Input: dimensioned drawing with shaded views. Units: mm. Origin: part minimum x, y, z. Coordinates: 2 decimals unless noted, no trailing zeros. Loops run counter-clockwise (first coordinate to the right, second up) from the corner with the lowest first, then second, coordinate; pieces in that order, holes last.
Item 1: Pull-direction query (X, two-part tool) for the marked faces 1, 2 and 3; classes: +X half, -X half, draft (parallel to the pull), parting line (faces both ways), or undercut.
Item 2: Line query: probe 1 along Y at (x, z) = (127.5, 7.25); probe 2 along Y at (x, z) = (75, 15.5); probe 3 along X at (y, z) = (50, 4). Output: solid intervals per line, ascending.
Item 3: Section query D-D, the plane y = 47.5. Return the cut outline in (x, z), then the cut area to 3 significant figures.
Item 4: Section query B-B, the plane y = 20. Return the cut outline in (x, z).
Item 5: Section query C-C, the plane z = 11.25. Return the cut outline in (x, y), then the cut area to 3 significant figures.
Item 6: Section query A-A, the plane x = 75. Return the cut outline in (y, z), then the cut area to 3 significant figures.
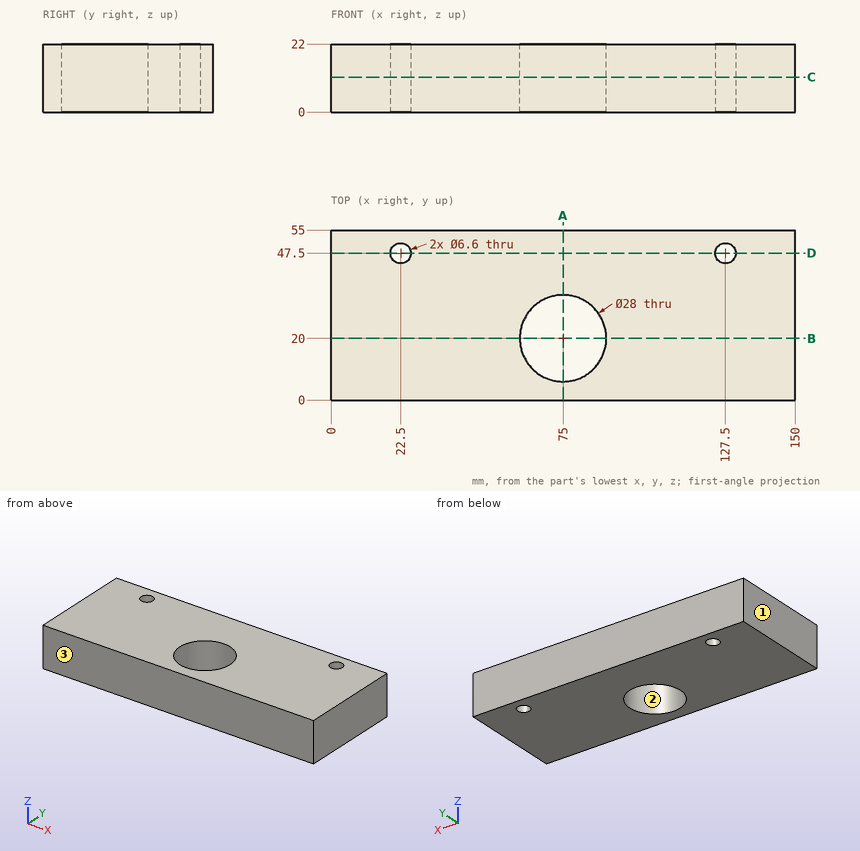
Verdict:
1. face 1: -X half
1. face 2: undercut
1. face 3: draft
2. probe 1: y = 0 to 44.2, 50.8 to 55
2. probe 2: y = 0 to 6, 34 to 55
2. probe 3: x = 0 to 20.35, 24.65 to 125.35, 129.65 to 150
3. outline: (0, 0) - (19.2, 0) - (19.2, 22) - (0, 22) - close; (25.8, 0) - (124.2, 0) - (124.2, 22) - (25.8, 22) - close; (130.8, 0) - (150, 0) - (150, 22) - (130.8, 22) - close
3. area: 3,010 mm2
4. outline: (0, 0) - (61, 0) - (61, 22) - (0, 22) - close; (89, 0) - (150, 0) - (150, 22) - (89, 22) - close
5. outline: (0, 0) - (150, 0) - (150, 55) - (0, 55) - close; hole circle Ø6.6 at (22.5, 47.5); hole circle Ø28 at (75, 20); hole circle Ø6.6 at (127.5, 47.5)
5. area: 7,570 mm2
6. outline: (0, 0) - (6, 0) - (6, 22) - (0, 22) - close; (34, 0) - (55, 0) - (55, 22) - (34, 22) - close
6. area: 594 mm2
